from build123d import *

# Parameters (mm, degrees)
SKETCH1_W           = 103
SKETCH1_H           = 83
BOSS_EXTRUDE1_DEPTH = 2
BOSS_EXTRUDE3_DEPTH = 2
CUT_EXTRUDE1_DEPTH  = 1
SKETCH5_W           = 1.778066781
SKETCH5_H           = 9.245947266
SKETCH5_W_2         = 1.778066782
CUT_EXTRUDE2_DEPTH  = 1


with BuildPart() as part:
    # Sketch1 → Boss-Extrude1 (new body)
    with BuildSketch(Plane.XY):
        with BuildLine():
            Line((-52.7, 42), (-52.7, -42))
            ThreePointArc((-52.7, -42), (-52.494974747, -42.494974747), (-52, -42.7))
            Line((-52, -42.7), (52, -42.7))
            ThreePointArc((52, -42.7), (52.494974747, -42.494974747), (52.7, -42))
            Line((52.7, -42), (52.7, 42))
            ThreePointArc((52.7, 42), (52.494974747, 42.494974747), (52, 42.7))
            Line((52, 42.7), (-52, 42.7))
            ThreePointArc((-52, 42.7), (-52.494974747, 42.494974747), (-52.7, 42))
        make_face()
        Rectangle(SKETCH1_W, SKETCH1_H, mode=Mode.SUBTRACT)
    extrude(amount=BOSS_EXTRUDE1_DEPTH)

    # Sketch3 → Boss-Extrude3 (add)
    with BuildSketch(Plane.XY.offset(2)):
        with BuildLine():
            Line((52, 45), (-52, 45))
            ThreePointArc((-52, 45), (-54.121320344, 44.121320344), (-55, 42))
            Line((-55, 42), (-55, -42))
            ThreePointArc((-55, -42), (-54.121320344, -44.121320344), (-52, -45))
            Line((-52, -45), (52, -45))
            ThreePointArc((52, -45), (54.121320344, -44.121320344), (55, -42))
            Line((55, -42), (55, 42))
            ThreePointArc((55, 42), (54.121320344, 44.121320344), (52, 45))
        make_face()
    extrude(amount=BOSS_EXTRUDE3_DEPTH)

    # Sketch4 → Cut-Extrude1 (cut)
    # profile 1 of 3: a face of its own
    with BuildSketch(Plane.XY.offset(4)):
        Polygon((12.961332904, 24.04515047), (-13.167559701, 24.04515047), (6.462349451, -9.95484953), (26.092258604, 24.04515047), align=None)
        Polygon((-6.239356471, 20.04515047), (6.033129674, 20.04515047), (19.164055373, 20.04515047), (6.462349451, -1.95484953), align=None, mode=Mode.SUBTRACT)
    # profile 2 of 3: a face of its own
    with BuildSketch(Plane.XY.offset(4)):
        Polygon((0.358766817, 10.216865701), (5.571249459, 19.24515047), (10.190051612, 19.24515047), (2.668167894, 6.216865701), align=None)
    # profile 3 of 3: a face of its own
    with BuildSketch(Plane.XY.offset(4)):
        Polygon((-14.091320132, 24.04515047), (-11.781919055, 20.04515047), (-19.37028217, 20.04515047), (-6.668576248, -1.95484953), (-2.874394691, 4.616865701), (-0.564993614, 0.616865701), (-6.668576248, -9.95484953), (-26.298485401, 24.04515047), align=None)
    extrude(amount=-CUT_EXTRUDE1_DEPTH, mode=Mode.SUBTRACT)

    # Sketch5 → Cut-Extrude2 (cut)
    with BuildSketch(Plane.XY.offset(4)):
        with Locations((-12.872296082, -17.930038178)):
            Rectangle(SKETCH5_W, SKETCH5_H)
        Polygon((-10.205195909, -22.553011811), (-10.205195909, -13.307064545), (-7.197299603, -13.307064545), (-5.641491169, -19.613645162), (-4.085682735, -13.307064545), (-1.077786429, -13.307064545), (-1.077786429, -22.553011811), (-2.85585321, -22.553011811), (-2.915122103, -15.274050923), (-4.650589368, -22.553011811), (-6.632392969, -22.553011811), (-8.367860234, -15.274050923), (-8.427129127, -22.553011811), align=None)
        Polygon((1.965300782, -22.553011811), (-0.24802193, -13.307064545), (1.574496521, -13.307064545), (3.01176717, -19.658096832), (4.532384699, -13.307064545), (6.958704995, -13.307064545), (8.464505301, -19.7655217), (9.898071644, -13.307064545), (11.724294401, -13.307064545), (9.551719052, -22.553011811), (7.349509256, -22.553011811), (5.738136235, -15.640777196), (4.084163698, -22.553011811), align=None)
        with Locations((13.561630075, -17.930038178)):
            Rectangle(SKETCH5_W_2, SKETCH5_H)
    extrude(amount=-CUT_EXTRUDE2_DEPTH, mode=Mode.SUBTRACT)


solid = part.part
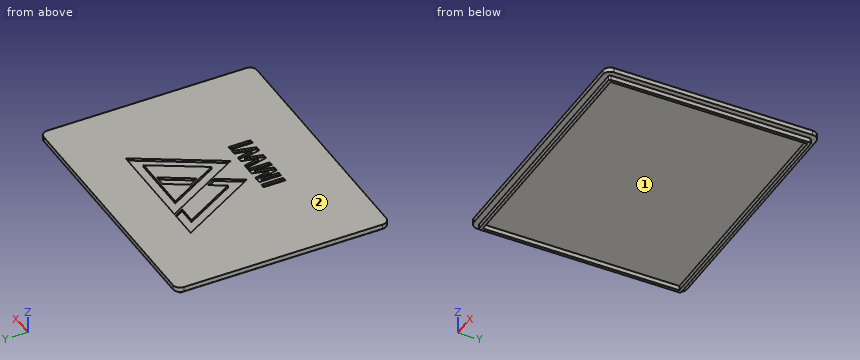
Part model, mm, in its own coordinate system. Face numbers are marked on the shaded views. Coordinates: 2 decimals unless noted, no trailing zeros. Order: outer loops, then holes, each group sorted by start corner. A loop starts at its lowest first (then second) coordinate and runs counter-clockwise, first axis right, second up. Notation, with made-up numbers: M -26,26 L 11,26 A13 cw 11,39 Z; hole C 87,11 d3. An arc over 180 degrees is marked long. One line per question, with ' | ' between items.
Q1. Slice it at C-C (x = -46.5). Give the cut face in (y, z), and give its area (3 significant figures).
A:
outline: M -45,2 L -42.7,2 L -42.7,0 L -41.5,0 L -41.5,2 L 41.5,2 L 41.5,0 L 42.7,0 L 42.7,2 L 45,2 L 45,4 L -45,4 Z | area: 185 mm^2
Q2. Slice it at A-A (y = -38). Give the cut face in (x, z), and give its area (3 significant figures).
A:
outline: M -55,2 L -52.7,2 L -52.7,0 L -51.5,0 L -51.5,2 L 51.5,2 L 51.5,0 L 52.7,0 L 52.7,2 L 55,2 L 55,4 L -55,4 Z | area: 225 mm^2
Q3. Slice it at B-B (z = 0.6). Give the cut face in (x, y).
A:
outline: M -52.7,-42 A0.7 ccw -52,-42.7 L 52,-42.7 A0.7 ccw 52.7,-42 L 52.7,42 A0.7 ccw 52,42.7 L -52,42.7 A0.7 ccw -52.7,42 Z; hole M -51.5,-41.5 L 51.5,-41.5 L 51.5,41.5 L -51.5,41.5 Z
Q4. Pin check, flat tips, straight feed: P1, Ø25, axis at x = -24.5, y = 9, coming from the -Z side; P2, Ø2, axis at x = 6, z = 0.5, coming from the -Y side; P3, Ø1, axis at x = -10, y = -17.5, coming from the +Z side; P4, Ø1, axis at y = -6, z = 1, coming from the -X side. Stop position of each tip, or through.
A:
P1: stops at z = 2 | P2: stops at y = -42.7 | P3: stops at z = 4 | P4: stops at x = -52.7
Q5. Two-plate mould, pull along X, no slides. Class the marked faces 1 and 2: +X half, -X half, draft (parallel to the pull), parting line (faces both ways), or undercut.
A:
face 1: undercut | face 2: draft
Q6. Slice it at D-D (y = -4). Give the cut face in (x, z), and give its area (3 significant figures).
A:
outline: M -55,2 L -52.7,2 L -52.7,0 L -51.5,0 L -51.5,2 L 51.5,2 L 51.5,0 L 52.7,0 L 52.7,2 L 55,2 L 55,4 L 9.9,4 L 9.9,3 L 3.02,3 L 3.02,4 L -3.23,4 L -3.23,3 L -10.11,3 L -10.11,4 L -55,4 Z | area: 211 mm^2
Q7. Drill centre lines: line 1 (Y direction, x = -2.5, z = 1.55); line 2 (X direction, y = 0, z = 1.1); line 3 (Z direction, x = -32, y = -3). Where is each one in solid material? Low to high.
A:
line 1: y = -42.7 to -41.5, 41.5 to 42.7 | line 2: x = -52.7 to -51.5, 51.5 to 52.7 | line 3: z = 2 to 4
